from build123d import *

# Parameters (mm, degrees)
ESQUISSE2_R             = 10
BOSS_EXTRU_1_DEPTH      = 7.5
ESQUISSE3_R             = 12
BOSS_EXTRU_2_DEPTH      = 7
ESQUISSE4_R             = 13.5
BOSS_EXTRU_3_DEPTH      = 1.5
ESQUISSE7_R             = 5.5
ENL_V_MAT_EXTRU_1_DEPTH = 21.5
ESQUISSE8_R             = 9
ENL_V_MAT_EXTRU_2_DEPTH = 7
CHANFREIN1_SIZE         = 0.7
ESQUISSE9_R             = 8
ENL_V_MAT_EXTRU_3_DEPTH = 1.25
ESQUISSE10_R            = 7
ENL_V_MAT_EXTRU_4_DEPTH = 3.5


with BuildPart() as part:
    # Esquisse2 → Boss.-Extru.1 (new body)
    with BuildSketch(Plane(origin=(0, 0, 0), x_dir=(1, 0, 0), z_dir=(0, 1, 0))):
        with Locations(Location((0, 0, 0), (0, 0, 270))):
            Circle(ESQUISSE2_R)
    extrude(amount=BOSS_EXTRU_1_DEPTH)

    # Esquisse3 → Boss.-Extru.2 (add)
    with BuildSketch(Plane(origin=(0, 7.5, 0), x_dir=(1, 0, 0), z_dir=(0, 1, 0))):
        with Locations(Location((0, 0, 0), (0, 0, 270))):
            Circle(ESQUISSE3_R)
    extrude(amount=BOSS_EXTRU_2_DEPTH)

    # Esquisse4 → Boss.-Extru.3 (add)
    with BuildSketch(Plane(origin=(0, 14.5, 0), x_dir=(1, 0, 0), z_dir=(0, 1, 0))):
        with Locations(Location((0, 0, 0), (0, 0, 270))):
            Circle(ESQUISSE4_R)
    extrude(amount=BOSS_EXTRU_3_DEPTH)

    # Esquisse7 → Enlèv. mat.-Extru.1 (cut)
    with BuildSketch(Plane.XZ):
        with Locations(Location((0, 0, 0), (0, 0, 270))):
            Circle(ESQUISSE7_R)
    extrude(amount=-ENL_V_MAT_EXTRU_1_DEPTH, mode=Mode.SUBTRACT)

    # Esquisse8 → Enlèv. mat.-Extru.2 (cut)
    with BuildSketch(Plane(origin=(0, 16, 0), x_dir=(1, 0, 0), z_dir=(0, 1, 0))):
        with Locations(Location((0, 0, 0), (0, 0, 270))):
            Circle(ESQUISSE8_R)
    extrude(amount=-ENL_V_MAT_EXTRU_2_DEPTH, mode=Mode.SUBTRACT)

    # Chanfrein1
    chanfrein1_edges = [part.edges().sort_by_distance(p)[0] for p in [
        (0, 16, -9),
    ]]
    chamfer(chanfrein1_edges, length=CHANFREIN1_SIZE)

    # Esquisse9 → Enlèv. mat.-Extru.3 (cut)
    with BuildSketch(Plane(origin=(0, 9, 0), x_dir=(1, 0, 0), z_dir=(0, 1, 0))):
        with Locations(Location((0, 0, 0), (0, 0, 270))):
            Circle(ESQUISSE9_R)
    extrude(amount=-ENL_V_MAT_EXTRU_3_DEPTH, mode=Mode.SUBTRACT)

    # Esquisse10 → Enlèv. mat.-Extru.4 (cut)
    with BuildSketch(Plane(origin=(0, 7.75, 0), x_dir=(1, 0, 0), z_dir=(0, 1, 0))):
        with Locations(Location((0, 0, 0), (0, 0, 270))):
            Circle(ESQUISSE10_R)
    extrude(amount=-ENL_V_MAT_EXTRU_4_DEPTH, mode=Mode.SUBTRACT)


solid = part.part
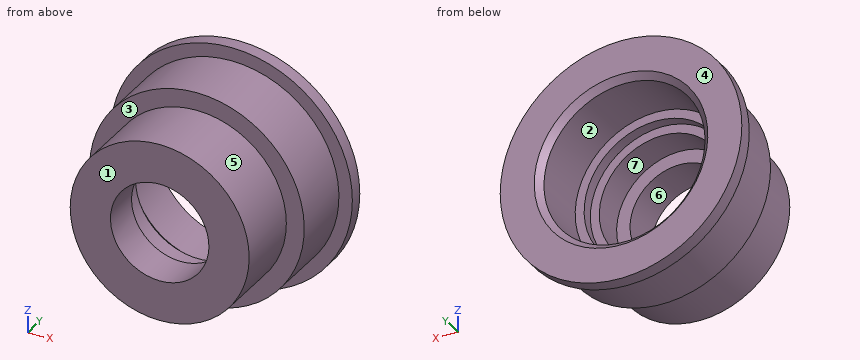
The model under review builds one solid part; all positions refer to its coordinate system, in mm. Face numbers are marked on the shaded views. A direction names the side the tool comes from. Coordinates: 2 decimals unless noted, no trailing zeros. Write each loop counter-clockwise with the first axis right and the second up, starting at its lowest first coordinate (ties: lowest second). Pieces come first, ordered by that corner, then holes. Notation, with made-up numbers: (34, -36) - (48, -36) arc R24 cw to (48, -5) - close; hole circle Ø2 at (7.25, 73.25). An arc over 180 degrees is marked (long way). Answer as a JSON object with one key per item and string values. Group by question number.
1. To check wall thickness, follow probe 1 along X at (y, z) = (8.1, 0); probe 2 along X at (y, z) = (11, 0); probe 3 along Y at (x, z) = (6, -4). State the ranges of each line that lie inside material, in increasing order.
2. Mouldability with a two-part tool opening along X and no side actions: class the marked faces 4, 5, 6 and 7 as pulls with the +X half, pulls with the -X half, needs draft (parallel to the pull), parting line crosses it, or undercut.
3. Add section C-C (y = 12.5). Give the boundary of the cut face in (x, z).
4. Clearance check with flat-ended pins moving along their axes: pin 1 Ø6 at (x, y) = (-4.5, 9) entering from -Z; pin 2 Ø9.5 at (x, z) = (0, 0) entering from -Y; pin 3 Ø5 at (x, z) = (-3.5, -1.5) entering from +Y; pin 4 Ø1 at (x, y) = (-1.5, 14.5) entering from -Z. State where each tip first meets the part, or that it passes through.
5. Machinability: for the marked faces 1, 2 and 3, which of the approach directions +Z, -Z, +X, -X, +Y, -Y give a long, thin tool a straight path to every point of the face, cutting with its end or side? Answer none if there is none.
6. Add section D-D (x = 11). Give the boundary of the cut face in (y, z), plus the area to 3 significant figures.
Findings:
{
 "1": {"probe 1": "-12 to -8, 8 to 12", "probe 2": "-12 to -9, 9 to 12", "probe 3": "0 to 7.75"},
 "2": {"face 4": "needs draft", "face 5": "parting line crosses it", "face 6": "undercut", "face 7": "undercut"},
 "3": {"outline": "circle Ø24 at (0, 0); hole circle Ø18 at (0, 0)"},
 "4": {"pin 1": "z = -11.91", "pin 2": "through", "pin 3": "y = 4.25", "pin 4": "z = -13.46"},
 "5": {"face 1": "+Z, -Z, +X, -X, -Y", "face 2": "+Y", "face 3": "-Y"},
 "6": {"outline": "(7.5, -4.8) - (14.5, -4.8) - (14.5, -7.83) - (16, -7.83) - (16, 7.83) - (14.5, 7.83) - (14.5, 4.8) - (7.5, 4.8) - close", "area": "90.6 mm²"}
}
